Part print with two shaded views. Sizes in mm from the minimum x, y, z corner. Round coordinates to 2 decimals unless told otherwise and drop trailing zeros. Write each loop counter-clockwise with the first axis right and the second up, starting at its lowest first coordinate (ties: lowest second). Pieces come first, ordered by that corner, then holes. Notation, with made-up numbers: (14.25, 61) -> (50.25, 61) arc R11 ccw to (50.25, 72) -> close; hole circle Ø11 at (89, 6.5). An arc over 180 degrees is marked (long way). Return JSON: item names as keys, results as strings. Group by question number.
(1) Drop a flat-ended pin along its axis: pin 1 Ø8 at (x, y) = (33, 7) entering from -Z. Give the stop position or say it passes through.
(2) Drill centre lines: L1, parallel to X at y = 12.5, z = 10; L2, parallel to X at y = 4, z = 9.5 (1 decimal); L3, parallel to X at y = 6.5, z = 17.5. Where is each one in solid material? Low to high. Write a range as from..to.
(3) Saw through at A-A (z = 10). List the corners of the cut face in (x, y), plus the area to 3 significant figures.
(4) Mould opens along X. For the marked faces 1, 2 and 3 say: +X half, -X half, draft (parallel to the pull), parting line (faces both ways), or undercut.
(5) Saw through at D-D (z = 32.5). List the corners of the cut face in (x, y).
(6) Saw through at C-C (x = 30). List the corners of the cut face in (y, z).
(7) Saw through at B-B (y = 3). List the corners of the cut face in (x, z) (1 decimal), plus the area to 3 significant figures.
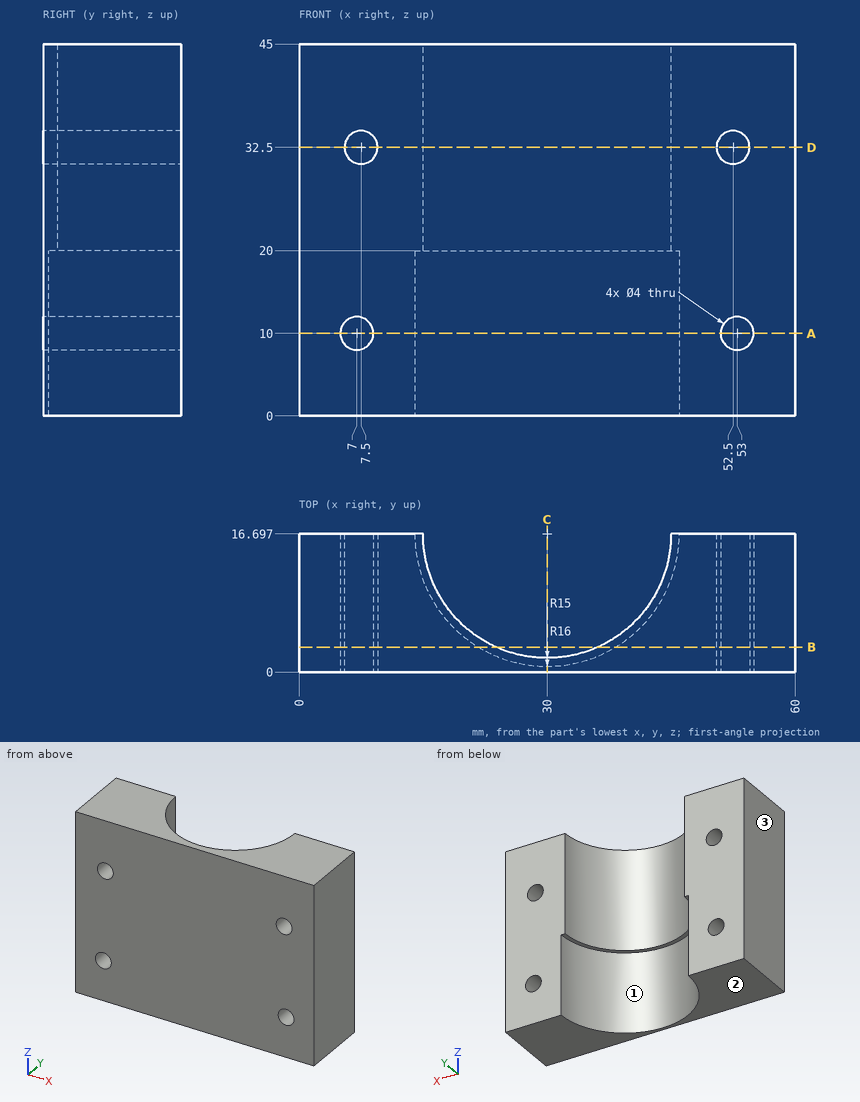
Computed values:
{
 "1": {"pin 1": "through"},
 "2": {"L1": "0..5, 9..14.56, 45.44..51, 55..60", "L2": "0..5.1, 8.9..20.3, 39.7..51.1, 54.9..60", "L3": "0..17.67, 42.33..60"},
 "3": {"outline": "(0, 0) -> (5, 0) -> (5, 16.7) -> (0, 16.7) -> close; (9, 0) -> (51, 0) -> (51, 16.7) -> (46, 16.7) arc R16 cw to (14, 16.7) -> (9, 16.7) -> close; (55, 0) -> (60, 0) -> (60, 16.7) -> (55, 16.7) -> close", "area": "466 mm2"},
 "4": {"face 1": "undercut", "face 2": "draft", "face 3": "-X half"},
 "5": {"outline": "(0, 0) -> (5.5, 0) -> (5.5, 16.7) -> (0, 16.7) -> close; (9.5, 0) -> (50.5, 0) -> (50.5, 16.7) -> (45, 16.7) arc R15 cw to (15, 16.7) -> (9.5, 16.7) -> close; (54.5, 0) -> (60, 0) -> (60, 16.7) -> (54.5, 16.7) -> close"},
 "6": {"outline": "(0, 0) -> (0.7, 0) -> (0.7, 20) -> (1.7, 20) -> (1.7, 45) -> (0, 45) -> close"},
 "7": {"outline": "(0, 0) -> (21.7, 0) -> (21.7, 20) -> (23.9, 20) -> (23.9, 45) -> (0, 45) -> close; (36.1, 20) -> (38.3, 20) -> (38.3, 0) -> (60, 0) -> (60, 45) -> (36.1, 45) -> close; hole circle Ø4 at (7, 10); hole circle Ø4 at (7.5, 32.5); hole circle Ø4 at (52.5, 32.5); hole circle Ø4 at (53, 10)", "area": "2,010 mm2"}
}
